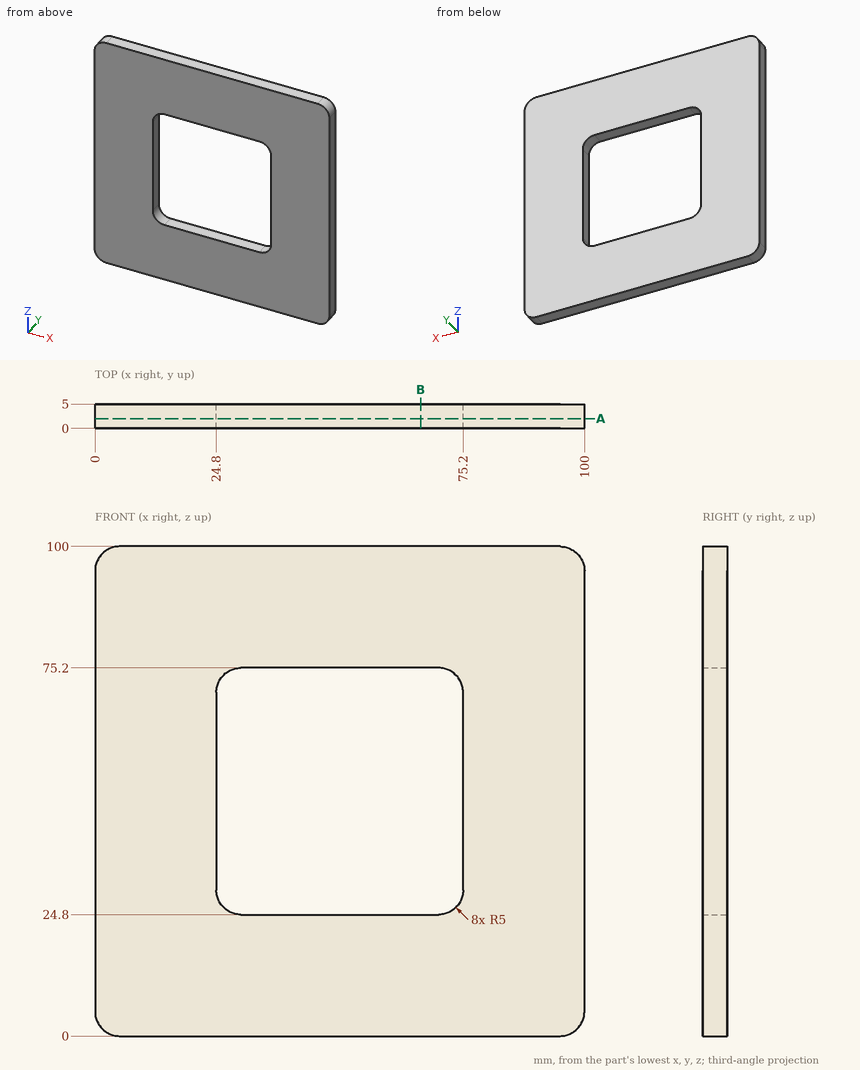
Drawing for the job (mm, zero at the part's lowest x, y, z). Round coordinates to 2 decimals unless told otherwise and drop trailing zeros. Loops run counter-clockwise (first coordinate to the right, second up) from the corner with the lowest first, then second, coordinate; pieces in that order, holes last. Notation, with made-up numbers: M 15.5,-18 L 47.5,-18 A8 ccw 47.5,-4 Z; hole C 38.5,46 d4. An arc over 180 degrees is marked long. Use a Markdown table: item, result. Add a question column.
(1) Cut at A-A (y = 2). Give the cut face in (x, z).
(2) Drill centre lines: line 1 (Z direction, x = 41, y = 4.3); line 2 (X direction, y = 4.6, z = 71). Where is each one in solid material? Low to high.
(3) Cut at B-B (x = 66.5). Give the cut face in (y, z).
Geometry says:
| question | item | result |
|---|---|---|
| 1 | outline | M 0,5 A5 ccw 5,0 L 95,0 A5 ccw 100,5 L 100,95 A5 ccw 95,100 L 5,100 A5 ccw 0,95 Z; hole M 24.8,29.8 A5 ccw 29.8,24.8 L 70.2,24.8 A5 ccw 75.2,29.8 L 75.2,70.2 A5 ccw 70.2,75.2 L 29.8,75.2 A5 ccw 24.8,70.2 Z |
| 2 | line 1 | z = 0 to 24.8, 75.2 to 100 |
| 2 | line 2 | x = 0 to 24.86, 75.14 to 100 |
| 3 | outline | M 0,0 L 5,0 L 5,24.8 L 0,24.8 Z; M 0,75.2 L 5,75.2 L 5,100 L 0,100 Z |
